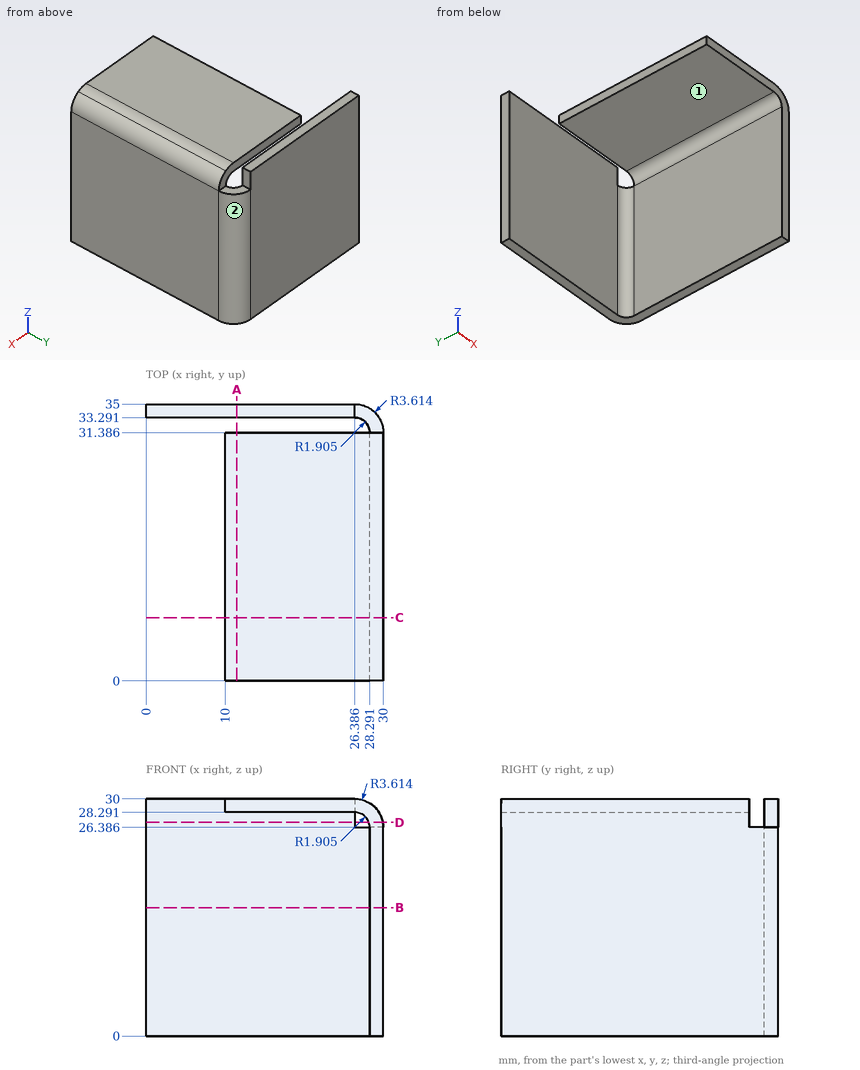
Check sheet for the drawn part. Datum: minimum x, y, z corner. Units: mm. A direction names the side the tool comes from. Round coordinates to 2 decimals unless told otherwise and drop trailing zeros. Order: outer loops, then holes, each group sorted by start corner. A loop starts at its lowest first (then second) coordinate and runs counter-clockwise, first axis right, second up.
(1) Go/stop test with flat-tipped pins: P1, Ø2, axis at x = 15, z = 16.5, coming from the -Y side; P2, Ø3, axis at x = 18.5, y = 17, coming from the -Z side; P3, Ø6, axis at y = 5.5, z = 22.5, coming from the -X side; P4, Ø8, axis at x = 16.5, y = 31, coming from the -Z side. Record where each tip stops, or that it passes through.
(2) Scan lines: probe 1 along Y at (x, z) = (16.5, 26.75); probe 2 along X at (y, z) = (19.5, 15). Record each from-to range of solid material in increasing order.
(3) Access from +Z, -Z, +X, -X, +Y, -Y to the whole of each face (thin tool, end or side, straight path). Record for the marked faces 1 and 2.
(4) Cross-section at B-B, the plane z = 16.25. Enter the section's corners in (x, y) (1 decimal), and give its area (3 significant figures).
(5) Cross-section at D-D, the plane z = 27. Enter the section's corners in (x, y) (1 decimal).
(6) Cross-section at A-A, the plane x = 11.5. Enter the section's corners in (y, z) (1 decimal).
(7) Cross-section at C-C, the plane y = 8. Enter the section's corners in (x, z) (1 decimal).
Check sheet entries:
1. P1: stops at y = 33.29
1. P2: stops at z = 28.29
1. P3: stops at x = 28.29
1. P4: stops at z = 0
2. probe 1: y = 33.29 to 35
2. probe 2: x = 28.29 to 30
3. face 1: -Z, -X, -Y
3. face 2: +Z, -Z, +X, +Y
4. outline: (0, 33.3) - (26.4, 33.3) arc R1.9 cw to (28.3, 31.4) - (28.3, 0) - (30, 0) - (30, 31.4) arc R3.6 ccw to (26.4, 35) - (0, 35) - close
4. area: 106 mm2
5. outline: (0, 33.3) - (26.4, 33.3) - (26.4, 35) - (0, 35) - close; (28.2, 0) - (29.9, 0) - (29.9, 31.4) - (28.2, 31.4) - close
6. outline: (0, 28.3) - (31.4, 28.3) - (31.4, 30) - (0, 30) - close; (33.3, 0) - (35, 0) - (35, 30) - (33.3, 30) - close
7. outline: (10, 28.3) - (26.4, 28.3) arc R1.9 cw to (28.3, 26.4) - (28.3, 0) - (30, 0) - (30, 26.4) arc R3.6 ccw to (26.4, 30) - (10, 30) - close
